Check sheet for the modelled part. Datum: model origin and axes. Units: mm. Coordinates: 2 decimals unless noted, no trailing zeros. Loops run counter-clockwise (first coordinate to the right, second up) from the corner with the lowest first, then second, coordinate; pieces in that order, holes last. Notation, with made-up numbers: (39, 68) -> (56, 68) arc R30 ccw to (56, 107) -> close; hole circle Ø6 at (21, 10.5). An arc over 180 degrees is marked (long way). Use CSV: the item, a comma, the result in double quotes.
```python
from build123d import *

# Parameters (mm, degrees)
LINEAR_AUSTRAGEN_D_NN1_DEPTH      = 170
LINEAR_AUSTRAGEN_D_NN1_DEPTH_BACK = 170
VERRUNDUNG1_R                     = 80
F_6_8_6_8_DURCHMESSER_BOHRUNG1_D  = 6.8


with BuildPart() as part:
    # Skizze2 → Linear-Austragen-Dünn1 (new body, two sides)
    with BuildSketch(Plane(origin=(0, 0, 0), x_dir=(1, 0, 0), z_dir=(0, 1, 0))) as linear_austragen_d_nn1_sk:
        with BuildLine():
            ThreePointArc((-169.777732917, -2.47495966), (0, -10), (169.777732917, -2.47495966))
            Line((169.777732917, -2.47495966), (170.662452734, -12.435746318))
            ThreePointArc((170.662452734, -12.435746318), (0, -20), (-170.662452734, -12.435746318))
            Line((-170.662452734, -12.435746318), (-169.777732917, -2.47495966))
        make_face()
    extrude(amount=LINEAR_AUSTRAGEN_D_NN1_DEPTH)
    extrude(linear_austragen_d_nn1_sk.sketch, amount=-LINEAR_AUSTRAGEN_D_NN1_DEPTH_BACK)

    # Verrundung1
    verrundung1_edges = [part.edges().sort_by_distance(p)[0] for p in [
        (170.220092826, 170, 7.455352989),
        (-170.220092826, 170, 7.455352989),
        (-170.220092826, -170, 7.455352989),
        (170.220092826, -170, 7.455352989),
    ]]
    fillet(verrundung1_edges, radius=VERRUNDUNG1_R)

    # Ø6.8 (6.8) Durchmesser Bohrung1 (through all)
    with Locations(Plane(origin=(-0.304533865, -134.419932379, 19.999975961), x_dir=(0.999999988, 0, 0.000157871), z_dir=(-0.000157871, 0, 0.999999988))):
        with Locations((0, 0)):
            Hole(F_6_8_6_8_DURCHMESSER_BOHRUNG1_D / 2)


solid = part.part
```
1) Thickness scan on line 1 along Z through (x, y) = (-14, -109.5); line 2 along Z through (x, y) = (49, -33); line 3 along X through (y, z) = (-122.5, 13). Record the ranges inside material, lowest first. Write a range as from..to.
Answer below:
line 1,"z = 9.95..19.95"
line 2,"z = 9.37..19.38"
line 3,"x = -163.79..163.79"
2) Cross-section at A-A on y = 59. Record the boundary of the cut face in (x, z), and give its area (3 significant figures).
Answer below:
outline,"(-170.66, 12.44) -> (-169.78, 2.47) arc R1919 cw to (169.78, 2.47) -> (170.66, 12.44) arc R1929 ccw to start"
area,"3,410 mm²"
3) Cross-section at B-B on x = 25.5. Record the boundary of the cut face in (y, z), and give its area (3 significant figures).
Answer below:
outline,"(-170, 9.83) -> (170, 9.83) -> (170, 19.83) -> (-170, 19.83) -> close"
area,"3,400 mm²"
4) Draft check along X on faces 1 (the flat face through (1, -170, 14)), 2 (the flat face through (-170.226, 1.26, 7.525)), 3 (the cylindrical face through (-2, 2, 10)). Enter one of: released by +X, released by -X, zero draft, split by the parting line, or undercut.
Answer below:
face 1,"zero draft"
face 2,"released by -X"
face 3,"undercut"
5) Go/stop test with flat-tipped pins: pin 1 Ø1 at (y, z) = (108.5, 9) entering from -X; pin 2 Ø5.5 at (x, y) = (-0.38, -134.42) entering from -Z. Record where each tip stops, or that it passes through.
Answer below:
pin 1,"stops at x = -168.31"
pin 2,"passes through"
